Design review of the part built by this model. Coordinates are the model's own, in mm. Face numbers are marked on the shaded views. A direction names the side the tool comes from. Give positions to 0.01 mm unless a question says otherwise; leave off trailing zeros. Loops run counter-clockwise (first coordinate to the right, second up) from the corner with the lowest first, then second, coordinate; pieces in that order, holes last. Notation, with made-up numbers: (-39.5, -13) -> (10.5, -13) arc R19 cw to (10.5, -9) -> close; hole circle Ø9 at (-12, -26). An arc over 180 degrees is marked (long way). Answer as CSV lines item,"result".
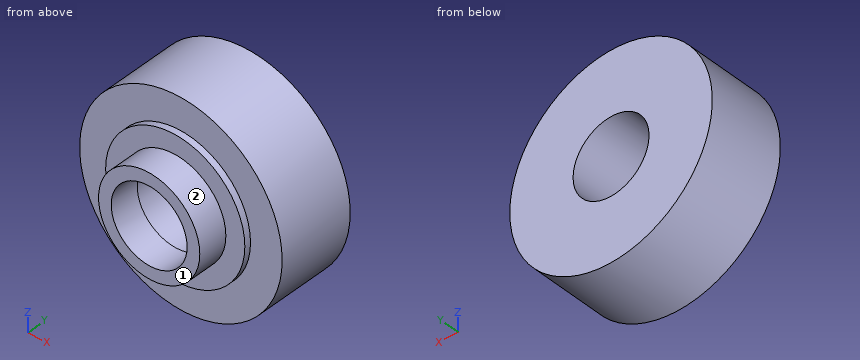
from build123d import *

# Parameters (mm, degrees)
F0_R      = 8
F1_DEPTH  = 6
F2_R      = 5.5
F3_DEPTH  = 0.5
F4_R      = 4
F4_R_2    = 3
F5_DEPTH  = 2.3
F5_FACE_R = 3
F6_DEPTH  = 6.501


with BuildPart() as f1:
    # F0 (on Front) → F1 (new body)
    with BuildSketch(Plane.XZ):
        Circle(F0_R)
    extrude(amount=F1_DEPTH)

    # F2 (on face) → F3 (join)
    with BuildSketch(Plane.XZ.offset(6)):
        Circle(F2_R)
    extrude(amount=F3_DEPTH)

    # F4 (on face) → F5 (join)
    with BuildSketch(Plane.XZ.offset(6.5)):
        Circle(F4_R)
        Circle(F4_R_2, mode=Mode.SUBTRACT)
    extrude(amount=F5_DEPTH)

    # F5_face (on face) → F6 (cut, through all)
    with BuildSketch(Plane.XZ.offset(6.5)):
        Circle(F5_FACE_R)
    extrude(amount=-F6_DEPTH, mode=Mode.SUBTRACT)


solid = f1.part
Q1. We need section C-C, the plane y = -7.5. State the section outline as (x, z) points.
Filled sheet:
outline,"circle Ø8 at (0, 0); hole circle Ø6 at (0, 0)"
Q2. We need section B-B, the plane x = 0. State the section outline as (y, z) points.
Filled sheet:
outline,"(-8.8, -4) -> (-6.5, -4) -> (-6.5, -5.5) -> (-6, -5.5) -> (-6, -8) -> (0, -8) -> (0, -3) -> (-8.8, -3) -> close; (-8.8, 3) -> (0, 3) -> (0, 8) -> (-6, 8) -> (-6, 5.5) -> (-6.5, 5.5) -> (-6.5, 4) -> (-8.8, 4) -> close"
Q3. We need section D-D, the plane z = -3.25. State the section outline as (x, y) points.
Filled sheet:
outline,"(-7.31, -6) -> (-4.44, -6) -> (-4.44, -6.5) -> (-2.33, -6.5) -> (-2.33, -8.8) -> (2.33, -8.8) -> (2.33, -6.5) -> (4.44, -6.5) -> (4.44, -6) -> (7.31, -6) -> (7.31, 0) -> (-7.31, 0) -> close"
Q4. Clearance check with flat-ended pins moving along their axes: pin 1 Ø5 at (x, y) = (4.5, -2) entering from +Z; pin 2 Ø4 at (x, y) = (-3, -3) entering from +Z; pin 3 Ø1.5 at (y, z) = (-4.5, -3) entering from +X. State where each tip first meets the part, or that it passes through.
Filled sheet:
pin 1,"stops at z = 7.75"
pin 2,"stops at z = 7.94"
pin 3,"stops at x = 7.68"
Q5. We need section A-A, the plane z = 0. State the section outline as (x, y) points.
Filled sheet:
outline,"(-8, -6) -> (-5.5, -6) -> (-5.5, -6.5) -> (-4, -6.5) -> (-4, -8.8) -> (-3, -8.8) -> (-3, 0) -> (-8, 0) -> close; (3, -8.8) -> (4, -8.8) -> (4, -6.5) -> (5.5, -6.5) -> (5.5, -6) -> (8, -6) -> (8, 0) -> (3, 0) -> close"
Q6. For the marked faces 1 and 2, list the 3-axis set-ups (+Z, -Z, +X, -X, +Y, -Y) from which the entire face can be reached by the end or side of a thin tool; tool diameter is ignored.
Filled sheet:
face 1,"+Z, -Z, +X, -X, -Y"
face 2,"-Y"
Q7. To check wall thickness, follow probe 1 along Z at (x, y) = (0, -3.75); probe 2 along Z at (x, y) = (0, -7); probe 3 along Y at (x, z) = (-5.75, 2.75). State the ranges of each line that lie inside material, in increasing order. Write a range as from..to.
Filled sheet:
probe 1,"z = -8..-3, 3..8"
probe 2,"z = -4..-3, 3..4"
probe 3,"y = -6..0"
